For this review, use the dimensioned drawing (mm, ordinates from the lowest corner) and the shaded views. A direction names the side the tool comes from. Coordinates: 2 decimals unless noted, no trailing zeros. Loops run counter-clockwise (first coordinate to the right, second up) from the corner with the lowest first, then second, coordinate; pieces in that order, holes last. Notation, with made-up numbers: (18, 76.25) - (74, 76.25) arc R33 cw to (74, 111.25) - close; hole circle Ø8 at (10, 1.5). An arc over 180 degrees is marked (long way). Use a Markdown table: item, result. Add a question column.
1) The part is to be moulded in two halves that separate along X. For the marked faces 3, 4 and 5, say which applies: pulls with the +X half, pulls with the -X half, needs draft (parallel to the pull), parting line crosses it, or undercut.
2) To check wall thickness, follow L1, parallel to Y at x = 5.9, z = 1.8; L2, parallel to Y at x = 36, z = 1.25; L3, parallel to X at y = 25, z = 4.2. State the ranges of each line that lie inside material, in increasing order. Write a range as [from, to].
3) Add section B-B, the plane y = 5.9. Give the boundary of the cut face in (x, z), and give its area (4 significant figures).
4) Add section D-D, the plane z = 1.5. Give the boundary of the cut face in (x, y), and give its area (3 significant figures).
5) Add section A-A, the plane x = 36.4. Give the boundary of the cut face in (y, z), and give its area (3 significant figures).
6) Clearance check with a flat-ended pin moving along its axis: pin 1 (5 mm diameter, centred on x = 36.4, y = 5.9, fed in from -Z). State where the tip first meets the part, or that it passes through.
7) For the marked faces 1 and 2, list the 3-axis set-ups (+Z, -Z, +X, -X, +Y, -Y) from which the entire face can be reached by the end or side of a thin tool; tool diameter is ignored.
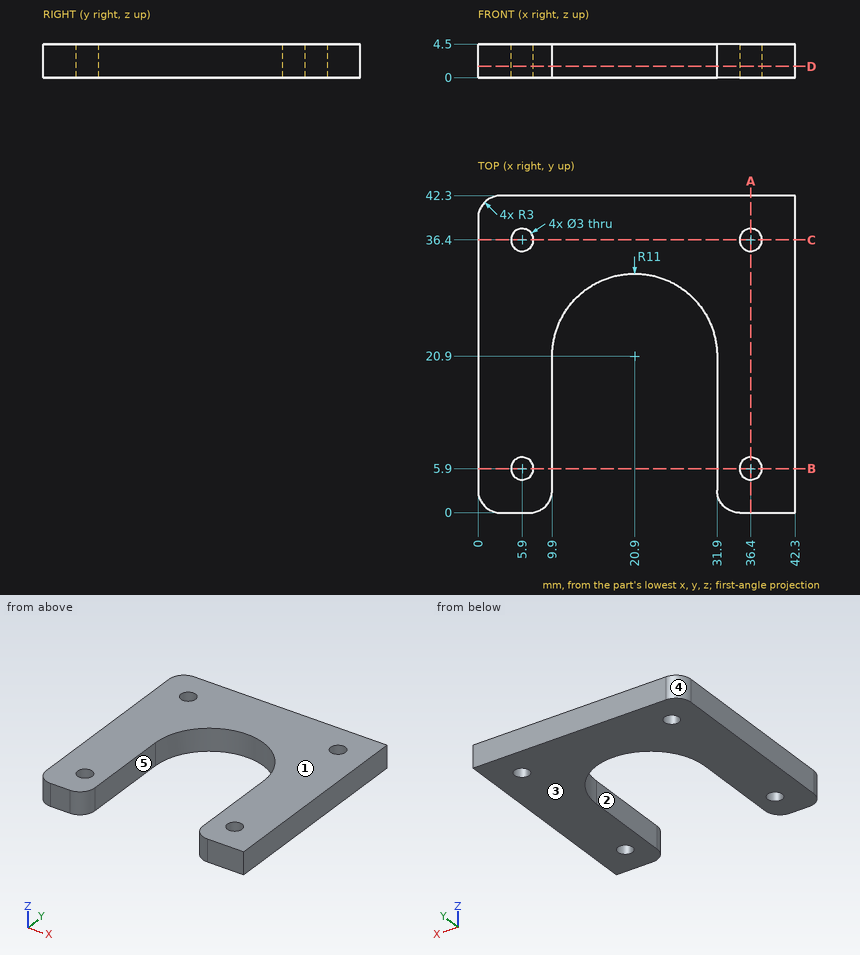
From the geometry:
| question | item | result |
|---|---|---|
| 1 | face 3 | needs draft |
| 1 | face 4 | pulls with the -X half |
| 1 | face 5 | undercut |
| 2 | L1 | y = [0, 4.4], [7.4, 34.9], [37.9, 42.3] |
| 2 | L2 | y = [0, 4.45], [7.35, 34.95], [37.85, 42.3] |
| 2 | L3 | x = [0, 10.69], [31.11, 42.3] |
| 3 | outline | (0, 0) - (4.4, 0) - (4.4, 4.5) - (0, 4.5) - close; (7.4, 0) - (9.9, 0) - (9.9, 4.5) - (7.4, 4.5) - close; (31.9, 0) - (34.9, 0) - (34.9, 4.5) - (31.9, 4.5) - close; (37.9, 0) - (42.3, 0) - (42.3, 4.5) - (37.9, 4.5) - close |
| 3 | area | 64.35 mm^2 |
| 4 | outline | (0, 3) arc R3 ccw to (3, 0) - (6.9, 0) arc R3 ccw to (9.9, 3) - (9.9, 20.9) arc R11 cw to (31.9, 20.9) - (31.9, 3) arc R3 ccw to (34.9, 0) - (42.3, 0) - (42.3, 42.3) - (3, 42.3) arc R3 ccw to (0, 39.3) - close; hole circle Ø3 at (5.9, 5.9); hole circle Ø3 at (5.9, 36.4); hole circle Ø3 at (36.4, 5.9); hole circle Ø3 at (36.4, 36.4) |
| 4 | area | 1,100 mm^2 |
| 5 | outline | (0, 0) - (4.4, 0) - (4.4, 4.5) - (0, 4.5) - close; (7.4, 0) - (34.9, 0) - (34.9, 4.5) - (7.4, 4.5) - close; (37.9, 0) - (42.3, 0) - (42.3, 4.5) - (37.9, 4.5) - close |
| 5 | area | 163 mm^2 |
| 6 | pin 1 | stops at z = 0 |
| 7 | face 1 | +Z, +X, -X, +Y, -Y |
| 7 | face 2 | +Z, -Z, -Y |
